For this review, take the finished solid that the model builds, in its own axes (mm). Face numbers are marked on the shaded views. Coordinates: 2 decimals unless noted, no trailing zeros. Loops run counter-clockwise (first coordinate to the right, second up) from the corner with the lowest first, then second, coordinate; pieces in that order, holes last.
1. Clearance check with flat-ended pins moving along their axes: P1, Ø20.5, axis at x = 20.5, y = 21.5, coming from the +Z side; P2, Ø1.5, axis at y = 8.5, z = 3.5, coming from the -X side; P3, Ø1.5, axis at x = 14, z = 1.5, coming from the +Y side; P4, Ø1, axis at y = 8, z = 1.5, coming from the -X side. State where each tip first meets the part, or that it passes through.
2. Take a section at A-A, the plane y = -23. State the section outline as (x, z) points, then the cut area to 3 significant figures.
3. To check wall thickness, follow probe 1 along X at (y, z) = (-0.5, 1); probe 2 along X at (y, z) = (7.5, 4.75); probe 3 along X at (y, z) = (7, 1.5). State the ranges of each line that lie inside material, in increasing order.
4. Take a section at D-D, the plane x = 0. State the section outline as (y, z) points, then the cut area to 3 significant figures.
5. Take a section at C-C, the plane y = 3.5. State the section outline as (x, z) points.
6. Take a section at B-B, the plane x = 10. State the section outline as (y, z) points.
7. Mouldability with a two-part tool opening along X and no side actions: class the marked faces 1, 2 and 3 as pulls with the +X half, pulls with the -X half, needs draft (parallel to the pull), parting line crosses it, or undercut.
```python
from build123d import *

# Parameters (mm, degrees)
F1_DEPTH = 7.0104
F2_D     = 22.060000076
F3_R     = 12.7
F4_DEPTH = 6.858
F5_R     = 12.7
F6_DEPTH = 6.858
F7_R     = 12.7
F8_DEPTH = 6.858
F9_D     = 22.060000076
F10_D    = 22.060000076
F11_D    = 22.060000076


with BuildPart() as f1:
    # F0 (on Top) → F1 (new body)
    with BuildSketch(Plane.XY):
        Polygon((15.2576936839, 25.2700417553), (-29.5133449568, 0.5785294558), (14.2556512728, -25.8485712111), align=None)
    extrude(amount=F1_DEPTH)

    # F2 (through all)
    with Locations(Plane(origin=(0, 0, 0), x_dir=(1, 0, 0), z_dir=(0, 0, -1))):
        with Locations((0, 0)):
            Hole(F2_D / 2)

    # F3 (on Top) → F4 (join)
    with BuildSketch(Plane.XY):
        with Locations((14.1001231968, -26.0360408574)):
            Circle(F3_R)
    extrude(amount=F4_DEPTH)

    # F5 (on Top) → F6 (join)
    with BuildSketch(Plane.XY):
        with Locations((15.4117625207, 25.3802221268)):
            Circle(F5_R)
    extrude(amount=F6_DEPTH)

    # F7 (on Top) → F8 (join)
    with BuildSketch(Plane.XY):
        with Locations((-29.4258532214, 0)):
            Circle(F7_R)
    extrude(amount=F8_DEPTH)

    # F9 (through all)
    with Locations(Plane(origin=(0, 0, 0), x_dir=(1, 0, 0), z_dir=(0, 0, -1))):
        with Locations((15.2576936839, -25.2700417553)):
            Hole(F9_D / 2)

    # F10 (through all)
    with Locations(Plane(origin=(0, 0, 0), x_dir=(1, 0, 0), z_dir=(0, 0, -1))):
        with Locations((14.2556512728, 25.8485712111)):
            Hole(F10_D / 2)

    # F11 (through all)
    with Locations(Plane(origin=(0, 0, 0), x_dir=(1, 0, 0), z_dir=(0, 0, -1))):
        with Locations((-29.5133449568, -0.5785294558)):
            Hole(F11_D / 2)


solid = f1.part
```
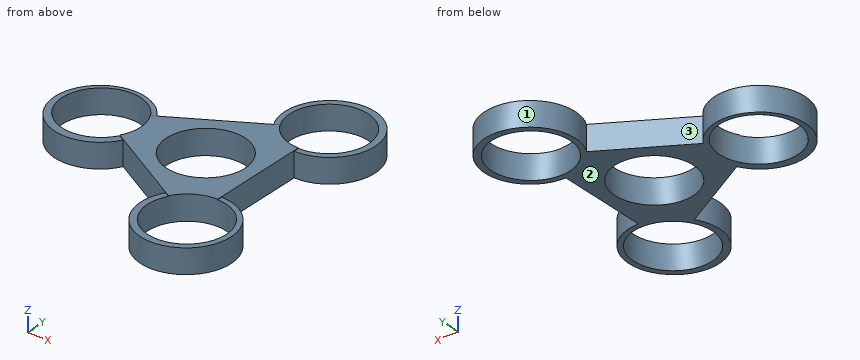
Results list:
1. P1: stops at z = 7.01
1. P2: stops at x = -39.49
1. P3: stops at y = 38.06
1. P4: stops at x = -39.67
2. outline: (1.77, 0) - (3.6, 0) - (3.6, 6.86) - (1.77, 6.86) - close; (24.91, 0) - (26.43, 0) - (26.43, 6.86) - (24.91, 6.86) - close
2. area: 23.0 mm2
3. probe 1: x = -42.12 to -40.49, -18.54 to -11.02, 11.02 to 14.75
3. probe 2: x = -39.67 to -38.1, -20.93 to -19.18, -16.96 to -8.09, 8.09 to 14.91
3. probe 3: x = -40.02 to -38.48, -20.55 to -18.83, -17.87 to -8.52, 8.52 to 14.9
4. outline: (-17.24, 0) - (-11.03, 0) - (-11.03, 7.01) - (-17.24, 7.01) - close; (11.03, 0) - (16.86, 0) - (16.86, 7.01) - (11.03, 7.01) - close
4. area: 84.4 mm2
5. outline: (-41.63, 0) - (-40.15, 0) - (-40.15, 6.86) - (-41.63, 6.86) - close; (-18.88, 0) - (-10.46, 0) - (-10.46, 7.01) - (-18.88, 7.01) - close; (10.46, 0) - (14.83, 0) - (14.83, 7.01) - (10.46, 7.01) - close
6. outline: (-38.06, 0) - (-36.02, 0) - (-36.02, 6.86) - (-38.06, 6.86) - close; (-15.67, 0) - (-4.65, 0) - (-4.65, 7.01) - (-15.67, 7.01) - close; (4.65, 0) - (15.57, 0) - (15.57, 7.01) - (4.65, 7.01) - close; (34.97, 0) - (36.87, 0) - (36.87, 6.86) - (34.97, 6.86) - close
7. face 1: parting line crosses it
7. face 2: needs draft
7. face 3: undercut
